Drawing for the job (mm, zero at the part's lowest x, y, z). A direction names the side the tool comes from. Give positions to 0.01 mm unless a question says otherwise; leave off trailing zeros. Order: outer loops, then holes, each group sorted by start corner. A loop starts at its lowest first (then second) coordinate and runs counter-clockwise, first axis right, second up. Notation, with made-up numbers: (36, 76.25) -> (49, 76.25) arc R16 cw to (49, 80.25) -> close; hole circle Ø3 at (63.5, 46). An arc over 180 degrees is marked (long way). One line per item, written item: value. Start each with the question number.
(1) Two-plate mould, pull along X, no slides. Class the marked faces 1, 2, 3 and 4: +X half, -X half, draft (parallel to the pull), parting line (faces both ways), or undercut.
(2) Saw through at A-A on y = 10. Give the cut face in (x, z).
(3) Probe line 1 (Y direction, x = 62.5, z = 5.25); line 2 (Z direction, x = 72, y = 8.5); line 3 (X direction, y = 6.75, z = 31) (1 decimal). List the from-to ranges inside material, lowest first.
(4) Which spindle directions (+Z, -Z, +X, -X, +Y, -Y) get a long thin tool onto all of the face, cutting with end or side? Do the marked faces 5 and 6. Say none if no direction does.
(5) Saw through at C-C on z = 4.5. Give the cut face in (x, y).
(6) Pin check, flat tips, straight feed: pin 1 (8 mm diameter, centred on x = 93.5, y = 9, fed in from +Z); pin 2 (2 mm diameter, centred on y = 10, z = 12.5, fed in from +X). Stop position of each tip, or through.
(7) Saw through at B-B on x = 62.5. Give the cut face in (y, z), plus the area to 3 significant figures.
(8) Saw through at D-D on z = 15. Give the cut face in (x, y), plus the area to 3 significant figures.
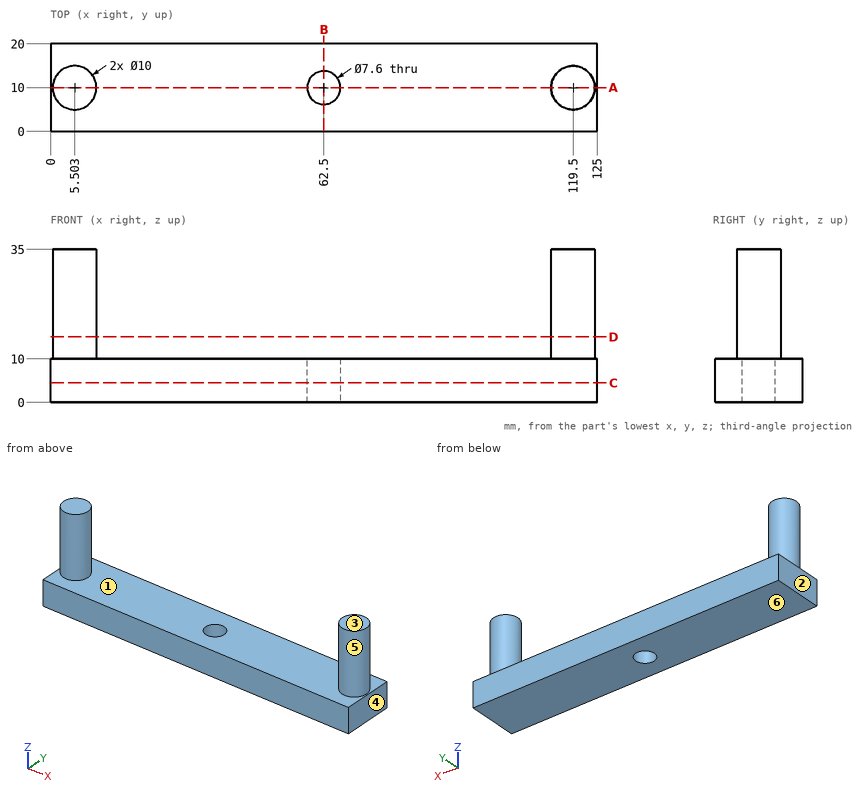
Results below:
1. face 1: undercut
1. face 2: -X half
1. face 3: draft
1. face 4: +X half
2. outline: (0, 0) -> (58.7, 0) -> (58.7, 10) -> (10.5, 10) -> (10.5, 35) -> (0.5, 35) -> (0.5, 10) -> (0, 10) -> close; (66.3, 0) -> (125, 0) -> (125, 10) -> (124.5, 10) -> (124.5, 35) -> (114.5, 35) -> (114.5, 10) -> (66.3, 10) -> close
3. line 1: y = 0 to 6.2, 13.8 to 20
3. line 2: z = 0 to 10
3. line 3: x = 1.7 to 9.3, 115.7 to 123.3
4. face 5: +Z
4. face 6: -Z, +X, -X, +Y, -Y
5. outline: (0, 0) -> (125, 0) -> (125, 20) -> (0, 20) -> close; hole circle Ø7.6 at (62.5, 10)
6. pin 1: stops at z = 10
6. pin 2: stops at x = 124.5
7. outline: (0, 0) -> (6.2, 0) -> (6.2, 10) -> (0, 10) -> close; (13.8, 0) -> (20, 0) -> (20, 10) -> (13.8, 10) -> close
7. area: 124 mm²
8. outline: circle Ø10 at (5.5, 10); circle Ø10 at (119.5, 10)
8. area: 157 mm²
